Build history of the part. All positions in model axes, mm. A direction names the side the tool comes from. Coordinates: 2 decimals unless noted, no trailing zeros. Loops run counter-clockwise (first coordinate to the right, second up) from the corner with the lowest first, then second, coordinate; pieces in that order, holes last.
Item 1: 3-axis set-ups, long thin cutter, end or side, ignore diameter. For faces 5 (the face through (-0.16, -0.49, -11.5)), 6 (the face through (-10.5, 1, 14)), 7 (the face through (0, -0.5, 0)), 8 (the face through (-6, 0, 4.4)), 9 (the face through (-0.76, -0.49, -1.28)): which of +Z, -Z, +X, -X, +Y, -Y reach the whole face in a straight line?
Item 2: Cut at A-A (x = -6). List the corners of the cut face in (y, z).
Item 3: Drill centre lines: line 1 along Z through (x, y) = (-6, -0.2); line 2 along X through (y, z) = (0.45, 13); line 3 along Y through (x, z) = (-7.75, 12). Where is each one in solid material? Low to high.
Item 4: Cut at C-C (z = -13.5). List the corners of the cut face in (x, y), and give its area (3 significant figures).
Item 5: Cut at D-D (x = 3.5). List the corners of the cut face in (y, z).
Item 6: Flat gauge pins, fed straight in: pin 1 (1 mm diameter, centred on x = 7.5, y = 1, fed in from -Z); pin 2 (1 mm diameter, centred on x = 6.5, y = 1.5, fed in from +Z); pin 3 (1 mm diameter, centred on x = -7, z = 9.5, fed in from -Y). Where does each tip first touch, or does it go through?
Item 7: Mould opens along Z. For faces 1 (the face through (-5, 1, 18.4)), 2 (the face through (6, 0, 4)), 3 (the face through (0.1, -0.5, -4)), 4 (the face through (-5, -1, 4)) say: released by +Z, released by -Z, zero draft, split by the parting line, or undercut.
Item 8: Cut at B-B (y = 0.4). List the corners of the cut face in (x, z).
from build123d import *

# Parameters (mm, degrees)
F1_DEPTH = 2.1
F4_DEPTH = 1
F7_DEPTH = 1
F2_R     = 1.5
F2_R_2   = 0.5
F8_DEPTH = 1


# Not quite as in the source:
# - a feature names something its author has since deleted; it is built from what else it names
# - the program builds the solid bodies; features that only make, move or delete a surface that nothing else refers to are left out


with BuildPart() as f1:
    # F0 (on Front) → F1 (new body)
    with BuildSketch(Plane.XZ):
        with BuildLine():
            ThreePointArc((-10.5, 9.2601295887), (-14, 0), (-10.5, -9.2601295887))
            Line((-10.5, -9.2601295887), (-10.5, -18.4))
            Line((-10.5, -18.4), (0, -18.4))
            Line((0, -18.4), (0, -15.3))
            Line((0, -15.3), (10.5, -15.3))
            Line((10.5, -15.3), (10.5, -9.2601295887))
            ThreePointArc((10.5, -9.2601295887), (14, 0), (10.5, 9.2601295887))
            Line((10.5, 9.2601295887), (10.5, 15.3))
            Line((10.5, 15.3), (0, 15.3))
            Line((0, 15.3), (0, 18.4))
            Line((0, 18.4), (-10.5, 18.4))
            Line((-10.5, 18.4), (-10.5, 9.2601295887))
        make_face()
    extrude(amount=-F1_DEPTH)

    # F3 (on face) → F4 (join)
    with BuildSketch(Plane.XZ):
        Polygon((1.5, 0), (-1.5, 0), (0, -2.5980762114), align=None)
    extrude(amount=F4_DEPTH)

    # F5 (on face) → F7 (join)
    with BuildSketch(Plane.XZ):
        with BuildLine():
            Line((0, -4), (-7.5, -4))
            ThreePointArc((-7.5, -4), (0, -11.5), (7.5, -4))
            Line((7.5, -4), (0, -4))
        make_face()
    extrude(amount=F7_DEPTH)

    # F2 (on Front) → F8 (join)
    with BuildSketch(Plane.XZ):
        with Locations((-6, 4.4)):
            Circle(F2_R)
        with Locations((-6, 4.4)):
            Circle(F2_R_2, mode=Mode.SUBTRACT)
        with Locations((5.9996811691, 4.3125251973)):
            Circle(F2_R)
        with Locations((5.9996811691, 4.3125251973)):
            Circle(F2_R_2, mode=Mode.SUBTRACT)
    extrude(amount=F8_DEPTH)


solid = f1.part
Filled sheet:
1. face 5: -Z, -Y
1. face 6: +Z, -X, +Y, -Y
1. face 7: +Z, +X, -X, -Y
1. face 8: -Y
1. face 9: -X, -Y
2. outline: (-1, -8.5) - (0, -8.5) - (0, -18.4) - (2.1, -18.4) - (2.1, 18.4) - (0, 18.4) - (0, 5.9) - (-1, 5.9) - (-1, 4.9) - (0, 4.9) - (0, 3.9) - (-1, 3.9) - (-1, 2.9) - (0, 2.9) - (0, -4) - (-1, -4) - close
3. line 1: z = -8.5 to -4, 2.9 to 3.9, 4.9 to 5.9
3. line 2: x = -10.5 to 10.5
3. line 3: y = 0 to 2.1
4. outline: (-10.5, 0) - (10.5, 0) - (10.5, 2.1) - (-10.5, 2.1) - close
4. area: 44.1 mm2
5. outline: (-1, -10.63) - (0, -10.63) - (0, -15.3) - (2.1, -15.3) - (2.1, 15.3) - (0, 15.3) - (0, -4) - (-1, -4) - close
6. pin 1: stops at z = -15.3
6. pin 2: stops at z = 15.3
6. pin 3: stops at y = 0
7. face 1: released by +Z
7. face 2: undercut
7. face 3: undercut
7. face 4: zero draft
8. outline: (-10.5, -18.4) - (0, -18.4) - (0, -15.3) - (10.5, -15.3) - (10.5, -9.26) arc R14 ccw to (10.5, 9.26) - (10.5, 15.3) - (0, 15.3) - (0, 18.4) - (-10.5, 18.4) - (-10.5, 9.26) arc R14 ccw to (-10.5, -9.26) - close
